```python
from build123d import *

# Parameters (mm, degrees)
F0_W     = 50.8
F0_H     = 25.4
F1_DEPTH = 12.7
F2_W     = 46.8
F2_H     = 23.4
F3_DEPTH = 25.4
F4_R     = 3
F5_R     = 1


with BuildPart() as f1:
    # F0 (on Front) → F1 (new body, symmetric)
    with BuildSketch(Plane.XZ):
        Rectangle(F0_W, F0_H)
    extrude(amount=F1_DEPTH, both=True)

    # F2 (on face) → F3 (cut, through all)
    with BuildSketch(Plane.XZ.offset(12.7)):
        with Locations((0, -1)):
            Rectangle(F2_W, F2_H)
    extrude(amount=-F3_DEPTH, mode=Mode.SUBTRACT)

    # F4
    f4_edges = [f1.edges().sort_by_distance(p)[0] for p in [
        (-25.4, 0, 12.7),
        (25.4, 0, 12.7),
    ]]
    fillet(f4_edges, radius=F4_R)

    # F5
    f5_edges = [f1.edges().sort_by_distance(p)[0] for p in [
        (-23.4, 0, 10.7),
        (23.4, 0, 10.7),
    ]]
    fillet(f5_edges, radius=F5_R)


solid = f1.part
```
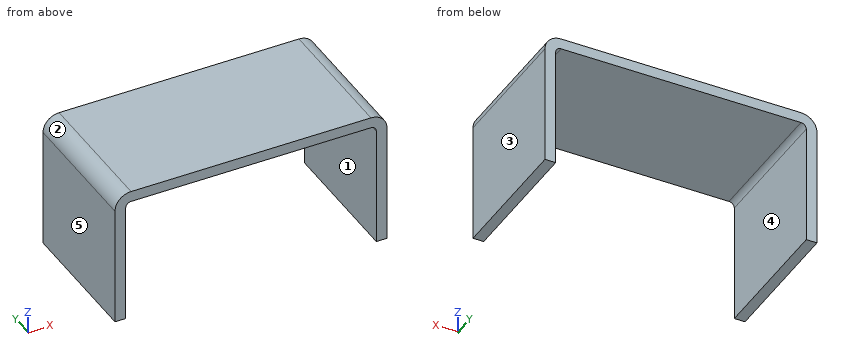
Model file for the job. Use its own axes, mm. Face numbers are marked on the shaded views. A direction names the side the tool comes from. Give positions to 0.01 mm unless a question says otherwise; leave off trailing zeros. Loops run counter-clockwise (first coordinate to the right, second up) from the corner with the lowest first, then second, coordinate; pieces in that order, holes last. Notation, with made-up numbers: M -4,-37 L 7,-37 A33 ccw 7,-6 Z; hole C 69.25,63 d8. An arc over 180 degrees is marked long. Use one line per item in the form item = value.
Item 1: Slice it at A-A on z = -3. List the corners of the cut face in (x, y), and give its area (3 significant figures).
Filled in:
outline = M -25.4,-12.7 L -23.4,-12.7 L -23.4,12.7 L -25.4,12.7 Z; M 23.4,-12.7 L 25.4,-12.7 L 25.4,12.7 L 23.4,12.7 Z
area = 102 mm^2
Item 2: Flat gauge pin, fed straight in: pin 1 Ø2 at (x, y) = (6.5, -0.5) entering from -Z. Where does the tip first touch, or does it go through?
Filled in:
pin_1 = 10.7
Item 3: Slice it at B-B on y = -3. List the corners of the cut face in (x, z).
Filled in:
outline = M -25.4,-12.7 L -23.4,-12.7 L -23.4,9.7 A1 cw -22.4,10.7 L 22.4,10.7 A1 cw 23.4,9.7 L 23.4,-12.7 L 25.4,-12.7 L 25.4,9.7 A3 ccw 22.4,12.7 L -22.4,12.7 A3 ccw -25.4,9.7 Z
Item 4: Slice it at C-C on x = 7.5. List the corners of the cut face in (y, z).
Filled in:
outline = M -12.7,10.7 L 12.7,10.7 L 12.7,12.7 L -12.7,12.7 Z
Item 5: Drill centre lines: L1, parallel to X at y = 5.25, z = -8.5; L2, parallel to Z at x = -5, y = -1.5; L3, parallel to X at y = -11, z = 11.25. Where is each one in solid material? Low to high.
Filled in:
L1 = -25.4 to -23.4, 23.4 to 25.4
L2 = 10.7 to 12.7
L3 = -24.97 to 24.97
Item 6: Which spindle directions (+Z, -Z, +X, -X, +Y, -Y) get a long thin tool onto all of the face, cutting with end or side? Do the marked faces 1 and 2. Say none if no direction does.
Filled in:
face_1 = -Z, +Y, -Y
face_2 = +Z, -X, +Y, -Y
Item 7: Two-plate mould, pull along X, no slides. Class the marked faces 3, 4 and 5: released by +X, released by -X, zero draft, split by the parting line, or undercut.
Filled in:
face_3 = released by +X
face_4 = undercut
face_5 = released by -X
